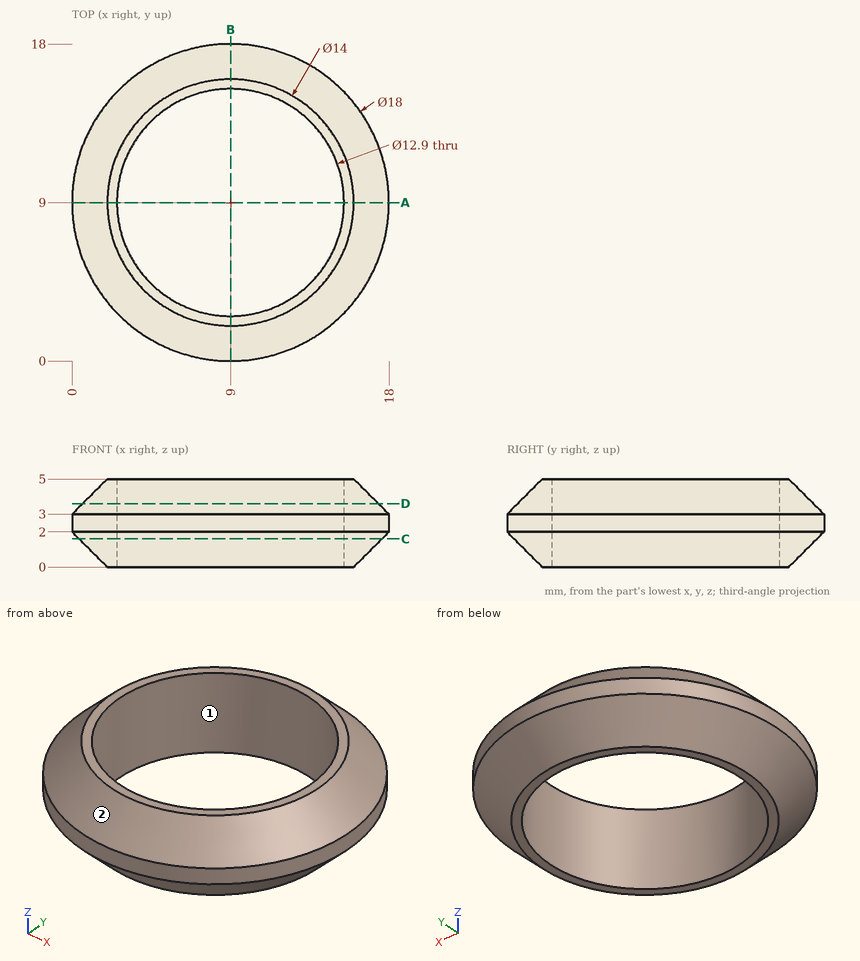
Part print with two shaded views. Sizes in mm from the minimum x, y, z corner. Coordinates: 2 decimals unless noted, no trailing zeros. Loops run counter-clockwise (first coordinate to the right, second up) from the corner with the lowest first, then second, coordinate; pieces in that order, holes last. Notation, with made-up numbers: M -8,85 L 31,85 A24 cw 31,100 Z; hole C 25.25,-13 d7. An arc over 180 degrees is marked long. Use CSV: the item, a comma, the result in double quotes. Start each with the question number.
1. Band-saw the part on D-D, the plane z = 3.6. List the corners of the cut face in (x, y), then the cut area to 3 significant figures.
2. Probe probe 1 along X at (y, z) = (10.5, 4.25); probe 2 along X at (y, z) = (12.5, 0.3); probe 3 along Y at (x, z) = (9, 3.9). List the from-to ranges inside material, lowest first. Write a range as [from, to].
3. Flat gauge pins, fed straight in: pin 1 (10.5 mm diameter, centred on x = 9, y = 9, fed in from -Z); pin 2 (1.5 mm diameter, centred on y = 6, z = 3.5, fed in from +X); pin 3 (1 mm diameter, centred on y = 11.5, z = 3, fed in from -X); pin 4 (3 mm diameter, centred on x = 12.5, z = 4, fed in from +Y). Where does each tip first touch, or does it go through?
4. Two-plate mould, pull along Y, no slides. Class the marked faces 1 and 2: pulls with the +Y half, pulls with the -Y half, needs draft (parallel to the pull), parting line crosses it, or undercut.
5. Band-saw the part on A-A, the plane y = 9. List the corners of the cut face in (x, z), then the cut area to 3 significant figures.
6. Band-saw the part on C-C, the plane z = 1.6. List the corners of the cut face in (x, y).
Entries:
1,outline,"C 9,9 d16.8; hole C 9,9 d12.9"
1,area,"91.0 mm2"
2,probe 1,"x = [1.4, 2.73], [15.27, 16.6]"
2,probe 2,"x = [2.59, 3.58], [14.42, 15.41]"
2,probe 3,"y = [0.9, 2.55], [15.45, 17.1]"
3,pin 1,"passes through"
3,pin 2,"stops at x = 17.66"
3,pin 3,"stops at x = 0.23"
3,pin 4,"stops at y = 17.68"
4,face 1,"undercut"
4,face 2,"parting line crosses it"
5,outline,"M 0,2 L 2,0 L 2.55,0 L 2.55,5 L 2,5 L 0,3 Z; M 15.45,0 L 16,0 L 18,2 L 18,3 L 16,5 L 15.45,5 Z"
5,area,"17.5 mm2"
6,outline,"C 9,9 d17.2; hole C 9,9 d12.9"
